Part model, mm, in its own coordinate system. A direction names the side the tool comes from. Give positions to 0.01 mm unless a question says otherwise; leave off trailing zeros. Order: outer loops, then holes, each group sorted by start corner. A loop starts at its lowest first (then second) coordinate and runs counter-clockwise, first axis right, second up. Notation, with made-up numbers: (79.5, -34.75) - (138.5, -34.75) arc R26 ccw to (138.5, 1.25) - close; hole circle Ø9 at (49.25, -34). An arc over 180 degrees is marked (long way). One line per item, written item: value.
```python
from build123d import *

# Parameters (mm, degrees)
HOLE_WIZARD_M31_D           = 3.4
HOLE_WIZARD_M31_CBORE_D     = 6.5
HOLE_WIZARD_M31_CBORE_DEPTH = 3
M3X0_51_D                   = 2.5
M3X0_51_DEPTH               = 15
M3X0_51_TIP                 = 0.751075774


with BuildPart() as part:
    # Эскиз2 → Повернуть1 (revolve)
    with BuildSketch(Plane(origin=(0, 0, 0), x_dir=(0, 0, -1), z_dir=(1, 0, 0)), mode=Mode.PRIVATE) as revolve_1_sk:
        Polygon((0, 0), (0, 16.5), (5, 16.5), (5, 6.3), (49, 6.3), (49, 0), align=None)
    revolve(revolve_1_sk.sketch.rotate(Axis((0, 0, -49), (0, 0, 1)), 90), axis=Axis((0, 0, -49), (0, 0, 1)))

    # Цековка для винта с внутренним шестигранником M31 (through all)
    with Locations(Plane.XY):
        with Locations((-12.5, 0), (0, 12.5), (12.5, 0), (0, -12.5)):
            CounterBoreHole(HOLE_WIZARD_M31_D / 2, HOLE_WIZARD_M31_CBORE_D / 2, HOLE_WIZARD_M31_CBORE_DEPTH)

    # Отверстие обработанное метчиком M3x0.51
    with Locations(Plane(origin=(2.706733298, -7.232806727, -49), x_dir=(-0.6355249951810988, -0.7720802940757291, 0), z_dir=(0, 0, -1))):
        with Locations((-3.864110878, 6.686444901)):
            Hole(M3X0_51_D / 2, depth=M3X0_51_DEPTH)
            with Locations((0, 0, -(M3X0_51_DEPTH + M3X0_51_TIP / 2))):  # 118° drill point
                Cone(0, M3X0_51_D / 2, M3X0_51_TIP, mode=Mode.SUBTRACT)


solid = part.part
```
1) Drill centre lines: line 1 along Y through (x, z) = (0, -4.35); line 2 along Y through (x, z) = (0, -37.5); line 3 along Z through (x, y) = (-2, 6.5). Where is each one in solid material? Low to high. Write a range as from..to.
Outcome:
line 1: y = -16.5..-14.2, -10.8..10.8, 14.2..16.5
line 2: y = -6.3..-1.25, 1.25..6.3
line 3: z = -5..0
2) Cut at A-A, the plane y = -12.5. Give the cut face in (x, z), then the cut area to 3 significant figures.
Outcome:
outline: (-10.77, -5) - (-1.7, -5) - (-1.7, -3) - (-3.25, -3) - (-3.25, 0) - (-10.77, 0) - close; (1.7, -5) - (10.77, -5) - (10.77, 0) - (3.25, 0) - (3.25, -3) - (1.7, -3) - close
area: 81.4 mm^2
3) Pin check, flat tips, straight feed: pin 1 (5 mm diameter, centred on x = 0, y = -12.5, fed in from +Z); pin 2 (5 mm diameter, centred on x = -1.5, y = -13, fed in from +Z); pin 3 (8 mm diameter, centred on x = -11.5, y = 8.5, fed in from -Z); pin 4 (8 mm diameter, centred on x = 4, z = -42.5, fed in from -Y). Stop position of each tip, or through.
Outcome:
pin 1: stops at z = -3
pin 2: stops at z = 0
pin 3: stops at z = -5
pin 4: stops at y = -6.3
4) Which spindle directions (+Z, -Z, +X, -X, +Y, -Y) get a long thin tool onto all of the face, cutting with end or side? Do faces 1 (the cylindrical face through (-15.738, -4.956, -2.535)), 2 (the cylindrical face through (-0.423, 15.722, -1.479)), 3 (the cylindrical face through (0.47, 1.16, -41.4)). Say none if no direction does.
Outcome:
face 1: +Z, -Z
face 2: +Z
face 3: -Z
5) Cut at B-B, the plane x = -13.5. Give the cut face in (y, z), then the cut area to 3 significant figures.
Outcome:
outline: (-9.49, -5) - (-1.37, -5) - (-1.37, -3) - (-3.09, -3) - (-3.09, 0) - (-9.49, 0) - close; (1.37, -5) - (9.49, -5) - (9.49, 0) - (3.09, 0) - (3.09, -3) - (1.37, -3) - close
area: 70.8 mm^2
6) Mould opens along Y. For faces 4 (the flat face through (1.4, -13.9, -3)), 5 (the flat face through (0, 7, -5)), 6 (the cylindrical face through (5, 3.83, -27.31)) say: released by +Y, released by -Y, zero draft, split by the parting line, or undercut.
Outcome:
face 4: undercut
face 5: zero draft
face 6: split by the parting line
7) Cut at C-C, the plane z = -19.5. Give the cut face in (x, y), then the cut area to 3 significant figures.
Outcome:
outline: circle Ø12.6 at (0, 0)
area: 125 mm^2
8) Cut at D-D, the plane y = -4.5. Give the cut face in (x, z), then the cut area to 3 significant figures.
Outcome:
outline: (-15.87, -5) - (-4.41, -5) - (-4.41, -49) - (4.41, -49) - (4.41, -5) - (15.87, -5) - (15.87, 0) - (-15.87, 0) - close
area: 547 mm^2
